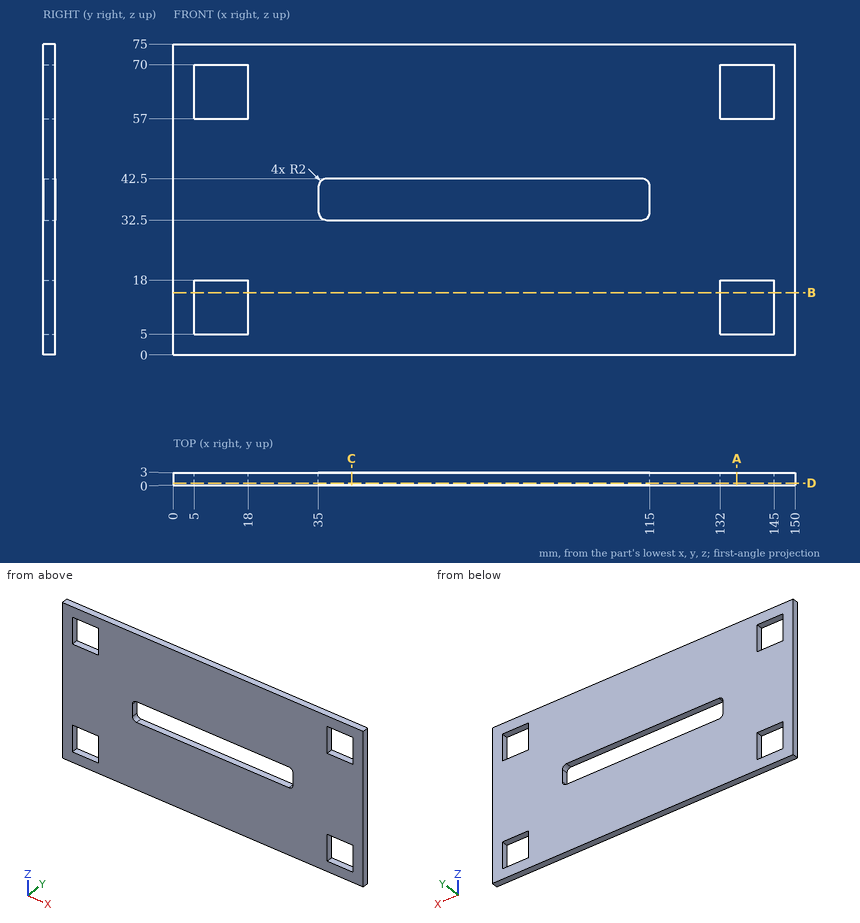
Job drawing, mm, ordinate dimensions from the low corner. One solid piece. Coordinates: 2 decimals unless noted, no trailing zeros. Write each loop counter-clockwise with the first axis right and the second up, starting at its lowest first coordinate (ties: lowest second). Pieces come first, ordered by that corner, then holes. Notation, with made-up numbers: (28, 73) -> (58, 73) arc R26 ccw to (58, 93) -> close; hole circle Ø11 at (-7, 16). An arc over 180 degrees is marked (long way). Use CSV: the item, a comma, the result in double quotes. Start each with the question number.
Item 1: Wall check: probe 1 along X at (y, z) = (0.85, 15); probe 2 along Z at (x, y) = (9, 0.2); probe 3 along Z at (x, y) = (82, 1). Give the ranges that are in metal, low to high.
Item 2: Band-saw the part on A-A, the plane x = 136. Write the cut outline in (y, z), plus the area to 3 significant figures.
Item 3: Band-saw the part on C-C, the plane x = 43. Write the cut outline in (y, z), plus the area to 3 significant figures.
Item 4: Band-saw the part on B-B, the plane z = 15. Write the cut outline in (x, y).
Item 5: Band-saw the part on D-D, the plane y = 0.5. Write the cut outline in (x, z), plus the area to 3 significant figures.
Response values:
1,probe 1,"x = 0 to 5, 18 to 132, 145 to 150"
1,probe 2,"z = 0 to 5, 18 to 57, 70 to 75"
1,probe 3,"z = 0 to 32.5, 42.5 to 75"
2,outline,"(0, 0) -> (3, 0) -> (3, 5) -> (0, 5) -> close; (0, 18) -> (3, 18) -> (3, 57) -> (0, 57) -> close; (0, 70) -> (3, 70) -> (3, 75) -> (0, 75) -> close"
2,area,"147 mm2"
3,outline,"(0, 0) -> (3, 0) -> (3, 32.5) -> (0, 32.5) -> close; (0, 42.5) -> (3, 42.5) -> (3, 75) -> (0, 75) -> close"
3,area,"195 mm2"
4,outline,"(0, 0) -> (5, 0) -> (5, 3) -> (0, 3) -> close; (18, 0) -> (132, 0) -> (132, 3) -> (18, 3) -> close; (145, 0) -> (150, 0) -> (150, 3) -> (145, 3) -> close"
5,outline,"(0, 0) -> (150, 0) -> (150, 75) -> (0, 75) -> close; hole (5, 5) -> (18, 5) -> (18, 18) -> (5, 18) -> close; hole (5, 57) -> (18, 57) -> (18, 70) -> (5, 70) -> close; hole (35, 34.5) arc R2 ccw to (37, 32.5) -> (113, 32.5) arc R2 ccw to (115, 34.5) -> (115, 40.5) arc R2 ccw to (113, 42.5) -> (37, 42.5) arc R2 ccw to (35, 40.5) -> close; hole (132, 5) -> (145, 5) -> (145, 18) -> (132, 18) -> close; hole (132, 57) -> (145, 57) -> (145, 70) -> (132, 70) -> close"
5,area,"9,780 mm2"
